from build123d import *

# Parameters (mm, degrees)
SKETCH_1_W               = 56.974706629
SKETCH_1_H               = 61.774716789
EXTRUDE_1_DEPTH          = 4
CUT_EXTRUDE_1_DEPTH      = 0.2
CUT_EXTRUDE_1_DEPTH_BACK = 2
SKETCH_2_W               = 4.870408941
SKETCH_2_H               = 4.364574549
SKETCH_2_H_2             = 4.39003302
SKETCH_2_W_2             = 4.274676149
SKETCH_2_H_3             = 2.486588773
SKETCH_3_W               = 10.898481077
SKETCH_3_H               = 8.614292609
CUT_EXTRUDE_2_DEPTH      = 3
SKETCH_4_W               = 9.753086106
SKETCH_4_H               = 5.329565659
CUT_EXTRUDE_3_DEPTH      = 2
SKETCH_5_R               = 1.5
SKETCH_5_R_2             = 1.35
CUT_EXTRUDE_4_DEPTH      = 2
SKETCH_6_W               = 3.227303784
SKETCH_6_H               = 21.254043688
CUT_EXTRUDE_5_DEPTH      = 2
SKETCH_7_R               = 1.55
SKETCH_7_R_2             = 1.3
SKETCH_7_R_3             = 0.9
SKETCH_7_W               = 3.1999746
SKETCH_7_H               = 1.7000254
CUT_EXTRUDE_8_DEPTH      = 3
SKETCH_9_W               = 4.274676149
SKETCH_9_H               = 2.586588773
SKETCH_9_W_2             = 5.070408941
SKETCH_9_H_2             = 4.471976124
SKETCH_9_H_3             = 4.444036068
CUT_EXTRUDE_9_DEPTH      = 2
SKETCH_10_W              = 35.063093726
SKETCH_10_H              = 2
CUT_EXTRUDE_10_DEPTH     = 47.363645154
EXTRUDE_2_DEPTH          = 1.5
SKETCH_12_R              = 1.8
CUT_EXTRUDE_11_DEPTH     = 5
SKETCH_13_R              = 3.8
CUT_EXTRUDE_12_DEPTH     = 1.5


with BuildPart() as part:
    # 草图1 → 凸台-拉伸1 (new body)
    with BuildSketch(Plane.XY):
        with Locations((3.938246432, -2.008964698)):
            Rectangle(SKETCH_1_W, SKETCH_1_H)
    extrude(amount=EXTRUDE_1_DEPTH)

    # 草图2 → 切除-拉伸1 (cut, two sides: drawn at the far end of the back side and taken through both)
    with BuildSketch(Plane(origin=(0, 0, 0), x_dir=(-1, 0, 0), z_dir=(0, 0, -1)).offset(-CUT_EXTRUDE_1_DEPTH_BACK)):
        with Locations((-11.822691441, 26.696106422)):
            Rectangle(SKETCH_2_W, SKETCH_2_H)
        with Locations((3.946198578, 26.683377186)):
            Rectangle(SKETCH_2_W, SKETCH_2_H_2)
        with Locations((4.061768809, 22.841086102)):
            Rectangle(SKETCH_2_W_2, SKETCH_2_H_3)
        with Locations((-11.938261672, 22.841086102)):
            Rectangle(SKETCH_2_W_2, SKETCH_2_H_3)
    extrude(amount=CUT_EXTRUDE_1_DEPTH + CUT_EXTRUDE_1_DEPTH_BACK, mode=Mode.SUBTRACT)

    # 草图3 → 切除-拉伸2 (cut)
    with BuildSketch(Plane(origin=(0, 0, 0), x_dir=(-1, 0, 0), z_dir=(0, 0, -1))):
        with Locations((-3.938246432, 24.571247392)):
            Rectangle(SKETCH_3_W, SKETCH_3_H)
    extrude(amount=-CUT_EXTRUDE_2_DEPTH, mode=Mode.SUBTRACT)

    # 草图4 → 切除-拉伸3 (cut)
    with BuildSketch(Plane(origin=(0, 0, 0), x_dir=(-1, 0, 0), z_dir=(0, 0, -1))):
        with Locations((-3.938246431, 17.599318258)):
            Rectangle(SKETCH_4_W, SKETCH_4_H)
    extrude(amount=-CUT_EXTRUDE_3_DEPTH, mode=Mode.SUBTRACT)

    # 草图5 → 切除-拉伸4 (cut)
    with BuildSketch(Plane(origin=(0, 0, 0), x_dir=(-1, 0, 0), z_dir=(0, 0, -1))):
        with Locations((-16.438279451, 21.841022601)):
            Circle(SKETCH_5_R)
        with Locations((-17.438279451, 24.341149602)):
            Circle(SKETCH_5_R_2)
        with Locations((-23.438279451, 21.841022601)):
            Circle(SKETCH_5_R)
        with Locations((-22.438279451, 24.341149602)):
            Circle(SKETCH_5_R_2)
        with Locations((8.561786589, 21.841022601)):
            Circle(SKETCH_5_R)
        with Locations((9.561786589, 24.341149602)):
            Circle(SKETCH_5_R_2)
        with Locations((15.561786589, 21.841022601)):
            Circle(SKETCH_5_R)
        with Locations((14.561786589, 24.341149602)):
            Circle(SKETCH_5_R_2)
    extrude(amount=-CUT_EXTRUDE_4_DEPTH, mode=Mode.SUBTRACT)

    # 草图6 → 切除-拉伸5 (cut)
    with BuildSketch(Plane(origin=(0, 0, 0), x_dir=(-1, 0, 0), z_dir=(0, 0, -1))):
        with Locations((20.935454991, 9.473060955)):
            Rectangle(SKETCH_6_W, SKETCH_6_H)
        with Locations((-28.811947854, 9.473058415)):
            Rectangle(SKETCH_6_W, SKETCH_6_H)
    extrude(amount=-CUT_EXTRUDE_5_DEPTH, mode=Mode.SUBTRACT)

    # 草图7 → 切除-拉伸8 (cut)
    with BuildSketch(Plane(origin=(0, 0, 0), x_dir=(-1, 0, 0), z_dir=(0, 0, -1))):
        with Locations((-1.438416122, -17.815866469)):
            Circle(SKETCH_7_R)
        with Locations((-6.438246431, -17.816005593)):
            Circle(SKETCH_7_R)
        with Locations((-9.438246431, -27.816005593)):
            Circle(SKETCH_7_R_2)
        with Locations((1.561753569, -27.816005593)):
            Circle(SKETCH_7_R_2)
        with Locations((11.054412954, -4.408667518)):
            Circle(SKETCH_7_R_3)
        with Locations((11.054412954, -9.408769118)):
            Circle(SKETCH_7_R_3)
        with Locations((11.804809195, -13.108944379)):
            Rectangle(SKETCH_7_W, SKETCH_7_H)
        with Locations((11.804809195, -17.908969779)):
            Rectangle(SKETCH_7_W, SKETCH_7_H)
        with Locations((11.804809195, -22.708969779)):
            Rectangle(SKETCH_7_W, SKETCH_7_H)
    extrude(amount=-CUT_EXTRUDE_8_DEPTH, mode=Mode.SUBTRACT)

    # 草图9 → 切除-拉伸9 (cut)
    with BuildSketch(Plane(origin=(0, 0, 0), x_dir=(-1, 0, 0), z_dir=(0, 0, -1))):
        with Locations((9.061778969, -26.409012958)):
            Rectangle(SKETCH_9_W, SKETCH_9_H)
        with Locations((8.946208738, -30.660335031)):
            Rectangle(SKETCH_9_W_2, SKETCH_9_H_2)
        with Locations((-16.938271831, -26.409012958)):
            Rectangle(SKETCH_9_W, SKETCH_9_H)
        with Locations((-16.822701601, -30.674305059)):
            Rectangle(SKETCH_9_W_2, SKETCH_9_H_3)
    extrude(amount=-CUT_EXTRUDE_9_DEPTH, mode=Mode.SUBTRACT)

    # 草图10 → 切除-拉伸10 (cut, through all)
    with BuildSketch(Plane(origin=(0, 0, 0), x_dir=(-1, 0, 0), z_dir=(0, 0, -1))):
        with Locations((-3.938119431, -31.896323093)):
            Rectangle(SKETCH_10_W, SKETCH_10_H)
    extrude(amount=-CUT_EXTRUDE_10_DEPTH, mode=Mode.SUBTRACT)

    # 草图11 → 凸台-拉伸2 (add)
    with BuildSketch(Plane(origin=(0, 0, 0), x_dir=(-1, 0, 0), z_dir=(0, 0, -1))):
        Polygon((6.381403048, 28.878393696), (24.549106883, 28.878393696), (24.549106883, -32.896323093), (13.593427432, -32.896323093), (13.593427432, -31.096323093), (14.493427432, -31.096323093), (14.493427432, -32.096323093), (23.749106883, -32.096323093), (23.749106883, -25.485957333), (22.749106883, -25.485957333), (22.749106883, -24.585957333), (23.749106883, -24.585957333), (23.749106883, -11.231931425), (22.749106883, -11.231931425), (22.749106883, -10.331931425), (23.749106883, -10.331931425), (23.749106883, 28.078393696), (17.038926543, 28.078393696), (17.038926543, 27.078393696), (16.138926543, 27.078393696), (16.138926543, 28.078393696), (7.981403048, 28.078393696), (7.981403048, 27.078393696), (6.381403048, 27.078393696), align=None)
        Polygon((-32.425599746, 28.878393696), (-32.425599746, -32.896323093), (-21.469666294, -32.896323093), (-21.469666294, -31.096323093), (-22.369666294, -31.096323093), (-22.369666294, -32.096323093), (-31.625599746, -32.096323093), (-31.625599746, -3.618963429), (-30.625599746, -3.618963429), (-30.625599746, 0.181036571), (-31.625599746, 0.181036571), (-31.625599746, 28.078393696), (-24.915165405, 28.078393696), (-24.915165405, 27.078393696), (-24.015165405, 27.078393696), (-24.015165405, 28.078393696), (-15.857895911, 28.078393696), (-15.857895911, 27.078393696), (-14.257895911, 27.078393696), (-14.257895911, 28.878393696), align=None)
    extrude(amount=EXTRUDE_2_DEPTH)

    # 草图12 → 切除-拉伸11 (cut)
    with BuildSketch(Plane(origin=(0, 0, 0), x_dir=(-1, 0, 0), z_dir=(0, 0, -1))):
        with Locations((19.561801829, 23.891088641)):
            Circle(SKETCH_12_R)
        with Locations((19.561801829, -27.909015499)):
            Circle(SKETCH_12_R)
        with Locations((-27.438294692, -27.909015499)):
            Circle(SKETCH_12_R)
        with Locations((-27.438294692, 23.891088641)):
            Circle(SKETCH_12_R)
    extrude(amount=-CUT_EXTRUDE_11_DEPTH, mode=Mode.SUBTRACT)

    # 草图13 → 切除-拉伸12 (cut)
    with BuildSketch(Plane.XY.offset(4)):
        with Locations((-19.561801829, -27.909015499)):
            Circle(SKETCH_13_R)
        with Locations((27.438294692, -27.909015499)):
            Circle(SKETCH_13_R)
        with Locations((27.438294692, 23.891088641)):
            Circle(SKETCH_13_R)
        with Locations((-19.561801829, 23.891088641)):
            Circle(SKETCH_13_R)
    extrude(amount=-CUT_EXTRUDE_12_DEPTH, mode=Mode.SUBTRACT)


solid = part.part
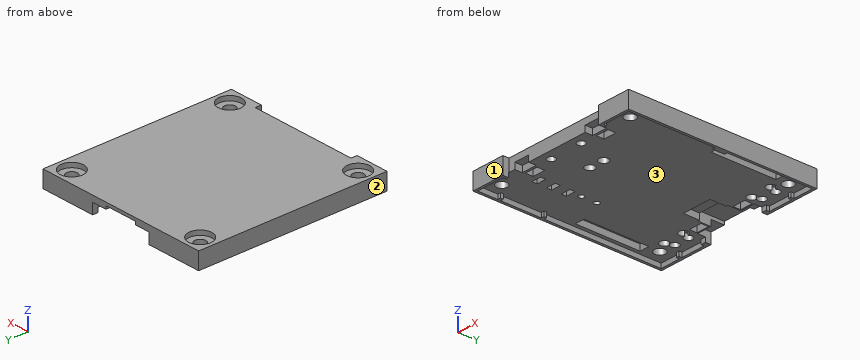
Part model, mm, in its own coordinate system. Face numbers are marked on the shaded views. Coordinates: 2 decimals unless noted, no trailing zeros. Write each loop counter-clockwise with the first axis right and the second up, starting at its lowest first coordinate (ties: lowest second). Pieces come first, ordered by that corner, then holes. Notation, with made-up numbers: (12.25, 7.25) - (18.25, 7.25) arc R36 cw to (18.25, 42.25) - close; hole circle Ø5 at (-23.75, 46.5). An arc over 180 degrees is marked (long way). Put each result on its own line as item: value.
1. Flat gauge pins, fed straight in: pin 1 Ø1.5 at (x, y) = (-2, 21.5) entering from -Z; pin 2 Ø2.5 at (x, y) = (29, 14.5) entering from -Z; pin 3 Ø1 at (x, z) = (-5, 0.5) entering from +Y; pin 4 Ø6 at (x, y) = (-18.5, -26) entering from +Z. Where does each tip first touch, or does it go through?
Final values:
pin 1: stops at z = 0
pin 2: stops at z = 2
pin 3: stops at y = 24.49
pin 4: stops at z = 4
2. Probe line 1 along X through (y, z) = (18, 1.95); line 2 along X through (y, z) = (12, 0.4); line 3 along Y through (x, z) = (27.5, 1.75). List the from-to ranges inside material, lowest first. Write a range as [from, to].
Final values:
line 1: x = [-24.55, -22.55], [-19.32, -0.94], [8.81, 27.2], [30.43, 32.43]
line 2: x = [-24.55, -22.55], [-19.32, 27.2], [30.43, 32.43]
line 3: y = [-32.9, -29.71], [-26.11, -1.15], [20.1, 22.09], [25.69, 28.88]
3. Band-saw the part on B-B (y = 18). Write the cut outline in (x, z), then the cut area to 3 significant figures.
Final values:
outline: (-24.55, -1.5) - (-23.75, -1.5) - (-23.75, 0) - (-22.55, 0) - (-22.55, 2) - (-19.32, 2) - (-19.32, 0) - (-0.94, 0) - (-0.94, 2) - (8.81, 2) - (8.81, 0) - (27.2, 0) - (27.2, 2) - (30.43, 2) - (30.43, 0) - (31.63, 0) - (31.63, -1.5) - (32.43, -1.5) - (32.43, 4) - (-24.55, 4) - close
area: 198 mm²
4. Band-saw the part on A-A (y = 6). Write the cut outline in (x, z), then the cut area to 3 significant figures.
Final values:
outline: (-24.55, -1.5) - (-23.75, -1.5) - (-23.75, 0) - (-22.55, 0) - (-22.55, 2) - (-19.32, 2) - (-19.32, 0) - (27.2, 0) - (27.2, 2) - (30.43, 2) - (30.43, 0) - (31.63, 0) - (31.63, -1.5) - (32.43, -1.5) - (32.43, 4) - (-24.55, 4) - close
area: 217 mm²
5. Two-plate mould, pull along Y, no slides. Class the marked faces 1, 2 and 3: +Y half, -Y half, draft (parallel to the pull), parting line (faces both ways), or undercut.
Final values:
face 1: -Y half
face 2: draft
face 3: undercut
6. Band-saw the part on C-C (z = 1.2). Give the number of separate pieces and of enclosed holes in the cut face, then the cut area to 3 significant figures.
Final values:
separate pieces: 1
enclosed holes: 23
area: 2,920 mm²
